The model under review builds one solid part; all positions refer to its coordinate system, in mm. Coordinates: 2 decimals unless noted, no trailing zeros. Write each loop counter-clockwise with the first axis right and the second up, starting at its lowest first coordinate (ties: lowest second). Pieces come first, ordered by that corner, then holes. Notation, with made-up numbers: (43, -29) - (54, -29) arc R15 ccw to (54, -8) - close; hole circle Ø1 at (-40, 45). An arc over 180 degrees is marked (long way). Answer as CSV lines item,"result". Start each with the question number.
Autodesk Inventor part; units mm, degrees
ref_plane "YZ Plane" through (0, 0, 0) normal (1, 0, 0) x (0, 1, 0)
ref_plane "XZ Plane" through (0, 0, 0) normal (0, 1, 0) x (-1, 0, 0)
ref_plane "XY Plane" through (0, 0, 0) normal (0, 0, 1) x (1, 0, 0)
sketch "Эскиз1" plane through (0, 0, 0) normal (0, 1, 0) x (-1, 0, 0)
  line L0 (-2.6795, -19) -> (83.0251, -19)
  line L1 (-2.6795, 244) -> (83.0251, 244)
  circle A0 centre (30.7479, 238.5) radius 1.85
  circle A1 centre (78.7479, 238.5) radius 1.85
  circle A2 centre (78.7479, -13.5) radius 1.85
  circle A3 centre (30.7479, -13.5) radius 1.85
  line L2 (83.0251, 244) -> (-2.6795, 244)
  line L3 (-2.6795, 244) -> (-2.6795, -19)
  line L4 (-2.6795, -19) -> (83.0251, -19)
  line L5 (83.0251, -19) -> (83.0251, 244)
  point P0 (0, 0)
  point P1 (83.0251, -19)
  point P2 (-2.6795, 244)
  dimension "d7" = 5.5
  dimension "d8" = 5.5
  dimension "d9" = 4.2772
  dimension "d10" = 48
  dimension "d11" = 263
  dimension "d12" = 5.5
  dimension "d13" = 5.5
  dimension "d14" = 4.2772
  dimension "d15" = 48
extrude "Выдавливание1" add sketch "Эскиз1" along normal blind 4
thicken "Толщина1" operation add thickness 2.671 both sides no extend neighbours yes toward (-1, 0, 0) faces at (2.6795, 1.3333, 156.3333)
sketch "Эскиз2" plane through (-1.399, 4, 60) normal (0, 1, 0) x (1, 0, 0)
  line L0 (-76.2625, -157.5) -> (-76.2625, 52.5)
  line L1 (-76.2625, 52.5) -> (-56.2625, 52.5)
  line L2 (-56.2625, -157.5) -> (-76.2625, -157.5)
  line L3 (-56.2625, 57.5) -> (-76.2625, 57.5)
  line L4 (-76.2625, 57.5) -> (-81.2625, 57.5)
  line L5 (-81.2625, 57.5) -> (-81.2625, -162.5)
  line L6 (-81.2625, -162.5) -> (-76.2625, -162.5)
  line L7 (-76.2625, -162.5) -> (-56.2625, -162.5)
  line L8 (-56.2625, -162.5) -> (-56.2625, -157.5)
  line L9 (-56.2625, 52.5) -> (-56.2625, 57.5)
  line L10 (1.4075, -184) -> (1.4075, 79)
  point P0 (0, 0)
  dimension "d21" = 57.67
  dimension "d22" = 25
  dimension "d23" = 5
extrude "Выдавливание2" cut sketch "Эскиз2" against normal blind 10
thicken "Толщина2" operation add thickness 2 both sides no extend neighbours yes toward (-1, 0, 0) faces at (-82.6615, 2.6667, 75.8333)
sketch "Эскиз3" plane through (0, 4, 0) normal (0, 1, 0) x (1, 0, 0)
  circle A0 centre (-51.7551, -83.34) radius 1.5
  circle A1 centre (-22.5451, -78.26) radius 1.5
  circle A2 centre (-22.5451, -127.79) radius 1.5
  circle A3 centre (-59.3751, -127.79) radius 1.5
  circle A4 centre (-22.2251, -142.53) radius 1.5
  circle A5 centre (-70.4851, -142.53) radius 1.5
  circle A6 centre (-22.2251, -214.92) radius 1.5
  circle A7 centre (-70.4851, -214.92) radius 1.5
  point P0 (0, 0)
extrude "Выдавливание3" cut sketch "Эскиз3" against normal blind 10
sketch "Эскиз4" plane through (0, 4, 0) normal (0, 1, 0) x (1, 0, 0)
  circle A0 centre (-19.9915, -174) radius 7.5
  line L0 (-83.0251, -244) -> (0.0085, -244)
  line L1 (0.0085, -244) -> (0.0085, 19)
  point P0 (0, 0)
  dimension "d26" = 15
  dimension "d27" = 70
  dimension "d28" = 20
extrude "Выдавливание4" cut sketch "Эскиз4" against normal blind 10
sketch "Эскиз5" plane through (0, 4, 0) normal (0, 1, 0) x (1, 0, 0)
  line L0 (-57.6615, -7.5) -> (-77.6615, -7.5)
  line L1 (-83.0251, -2.5) -> (-57.6615, -2.5)
  point P0 (0, 0)
  dimension "d31" = 5
properties part number "KB33-046-004-002 - Передняя пластина" material "Дерево (вишня)"
(1) Add section C-C on z = 118. Give the boundary of the cut face in (x, y).
(2) For pin 1 (3 mm diameter, centred on x = -78.75, z = 238.5, fed in from -Y), flat-tipped, find the tip position at first contact; note if it passes through.
(3) Wall thickness on line 1 (Z direction, x = -64.5, y = 1.1); line 2 (X direction, y = 1.1, z = 238.5); line 3 (Z direction, x = -31, y = 3.05): over which ranges is each line inside the solid? List them lowest first.
(4) Add section A-A on y = 3.2. Give the number of separate pieces and of enclosed holes in the cut face, then the cut area to 3 significant figures.
(5) Add section B-B on z = 170. Give the boundary of the cut face in (x, y).
(6) The part is to be moulded in two halves that separate along Z. For faces 1 (the cylindrical face through (-20.968, 2.028, 166.564)), 2 (the flat face through (-41, 0, 114)), say which applies: released by +Z, released by -Z, zero draft, split by the parting line, or undercut.
Reported:
1,outline,"(-77.66, 0) - (0.01, 0) - (0.01, 4) - (-77.66, 4) - close"
2,pin 1,"through"
3,line 1,"-19 to 2.5, 7.5 to 217.5, 222.5 to 244"
3,line 2,"-83.03 to -80.6, -76.9 to -32.6, -28.9 to 0.01"
3,line 3,"-19 to -15.33, -11.67 to 236.67, 240.33 to 244"
4,separate pieces,"1"
4,enclosed holes,"13"
4,area,"20,200 mm²"
5,outline,"(-77.66, 0) - (-26.34, 0) - (-26.34, 4) - (-77.66, 4) - close; (-13.65, 0) - (0.01, 0) - (0.01, 4) - (-13.65, 4) - close"
6,face 1,"undercut"
6,face 2,"zero draft"
